The model under review builds one solid part; all positions refer to its coordinate system, in mm. Coordinates: 2 decimals unless noted, no trailing zeros. Put each result on its own line as item: value.
from build123d import *

# Parameters (mm, degrees)
F0_W     = 71.032305
F0_H     = 3.316156
F0_W_2   = 70.65738
F0_H_2   = 4.029283
F0_W_3   = 70.945185
F0_H_3   = 4.029279
F0_W_4   = 71.23299
F0_H_4   = 3.453669
F0_W_5   = 71.426928
F0_H_5   = 3.551615
F0_W_6   = 72.216179
F0_H_6   = 3.354305
F0_W_7   = 72.610803
F0_H_7   = 2.762366
F0_W_8   = 73.005423
F0_H_8   = 3.354303
F0_W_9   = 72.808113
F0_H_9   = 3.354299
F1_DEPTH = 3.81


with BuildPart() as f1:
    # F0 (on Front) → F1 (new body)
    with BuildSketch(Plane.XZ):
        Polygon((56.841634, 59.431892), (-61.265364, 59.431892), (-61.265364, 47.354873), (-8.385758, 47.354873), (-8.385758, 44.197883), (-61.265364, 44.197883), (-61.265364, 36.305401), (-8.385758, 36.305401), (-8.385758, 33.345722), (-61.265364, 33.345722), (-61.265364, 25.847867), (-7.991134, 25.847867), (-7.991134, 22.888189), (-61.265364, 22.888189), (-61.265364, 14.798397), (-7.596511, 14.798397), (-7.793822, 11.246782), (-61.265364, 11.246782), (-61.265364, 3.597572), (-8.202464, 3.597572), (-8.202464, 0), (-61.265364, 0), (-61.265364, -9.641493), (-7.914659, -9.641493), (-7.914659, -13.382968), (-61.265364, -13.382968), (-61.265364, -24.031783), (-7.914659, -24.031783), (-7.914659, -27.485449), (-61.265364, -27.485449), (-61.265364, -38.134262), (-8.202464, -38.134262), (-8.202464, -42.163543), (-61.265364, -42.163543), (-61.265364, -53.076919), (-8.202464, -53.076919), (-8.202464, -55.690415), (-61.265364, -55.690415), (-61.265364, -69.217287), (56.841634, -69.217287), (56.841634, -56.036595), (11.206436, -56.036595), (11.206436, -53.076919), (56.841634, -53.076919), (56.841634, -42.163543), (11.206436, -42.163543), (11.080521, -38.134262), (56.841634, -38.134262), (56.841634, -28.348867), (6.475631, -28.348867), (6.475631, -24.031783), (56.841634, -24.031783), (56.841634, -13.382968), (6.475631, -13.382968), (6.475631, -9.641493), (56.841634, -9.641493), (56.841634, 0), (6.763437, 0), (6.475631, 3.597572), (56.841634, 3.597572), (56.841634, 11.444095), (6.412639, 11.444095), (6.412639, 14.798397), (56.841634, 14.798397), (56.841634, 22.690875), (6.215328, 22.690875), (6.215328, 25.847867), (56.841634, 25.847867), (56.841634, 33.345722), (6.215328, 33.345722), (6.215328, 36.305401), (56.841634, 36.305401), (56.841634, 44.000566), (6.018014, 44.000566), (6.018014, 47.354873), (56.841634, 47.354873), align=None)
        with Locations((0.690593, -47.27529)):
            Rectangle(F0_W, F0_H, mode=Mode.SUBTRACT)
        with Locations((0.50313, -33.241566)):
            Rectangle(F0_W_2, F0_H_2, mode=Mode.SUBTRACT)
        with Locations((0.647033, -19.714693)):
            Rectangle(F0_W_3, F0_H_3, mode=Mode.SUBTRACT)
        with Locations((0.790935, -4.173183)):
            Rectangle(F0_W_4, F0_H_4, mode=Mode.SUBTRACT)
        with Locations((0.887904, 7.695167)):
            Rectangle(F0_W_5, F0_H_5, mode=Mode.SUBTRACT)
        with Locations((0.690593, 18.448668)):
            Rectangle(F0_W_6, F0_H_6, mode=Mode.SUBTRACT)
        with Locations((0.887905, 29.202171)):
            Rectangle(F0_W_7, F0_H_7, mode=Mode.SUBTRACT)
        with Locations((1.085214, 40.350296)):
            Rectangle(F0_W_8, F0_H_8, mode=Mode.SUBTRACT)
        with Locations((0.98656, 51.202455)):
            Rectangle(F0_W_9, F0_H_9, mode=Mode.SUBTRACT)
    extrude(amount=F1_DEPTH)


solid = f1.part
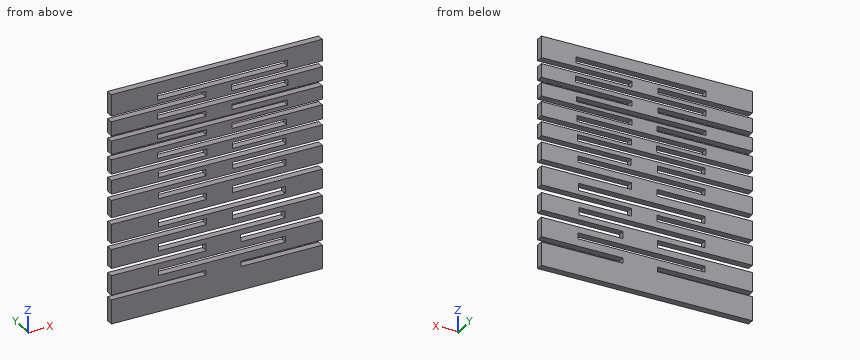
Item 1: Consider section A-A on x = 44. Count the separate pieces of the cut face and the enclosed holes in it, and give its area (3 significant figures).
Answers below:
separate pieces: 10
enclosed holes: 0
area: 370 mm^2
Item 2: For pin 1 Ø2 at (x, z) = (1.5, -14) entering from +Y; pin 2 Ø1.9 at (y, z) = (-1.5, -12) entering from +X; pin 3 Ø1.9 at (y, z) = (-1.5, -12) entering from -X, all flat-tipped, find the tip position at first contact; note any pin that passes through.
Answers below:
pin 1: y = 0
pin 2: x = 6.48
pin 3: x = -7.91
Item 3: For line 1 (X direction, y = -1.5, z = 40); line 2 (X direction, y = -0.9, z = -27); line 3 (X direction, y = -0.9, z = -46), list the stretches that pass through material, from the lowest coordinate up. Write a range as from..to.
Answers below:
line 1: -61.27..-35.42, 37.59..56.84
line 2: -7.91..6.48
line 3: -61.27..-34.83, 36.21..56.84
